Source: three-view drawing plus pictorial views. Frame: mm from the lowest corner of the part. Give positions to 0.01 mm unless a question says otherwise; leave off trailing zeros. Loops run counter-clockwise (first coordinate to the right, second up) from the corner with the lowest first, then second, coordinate; pieces in that order, holes last. Notation, with made-up numbers: (6.25, 35.5) - (24.25, 35.5) arc R33 ccw to (24.25, 73.5) - close; hole circle Ø1 at (45, 25.5). An arc over 180 degrees is marked (long way). One line per item, written item: value.
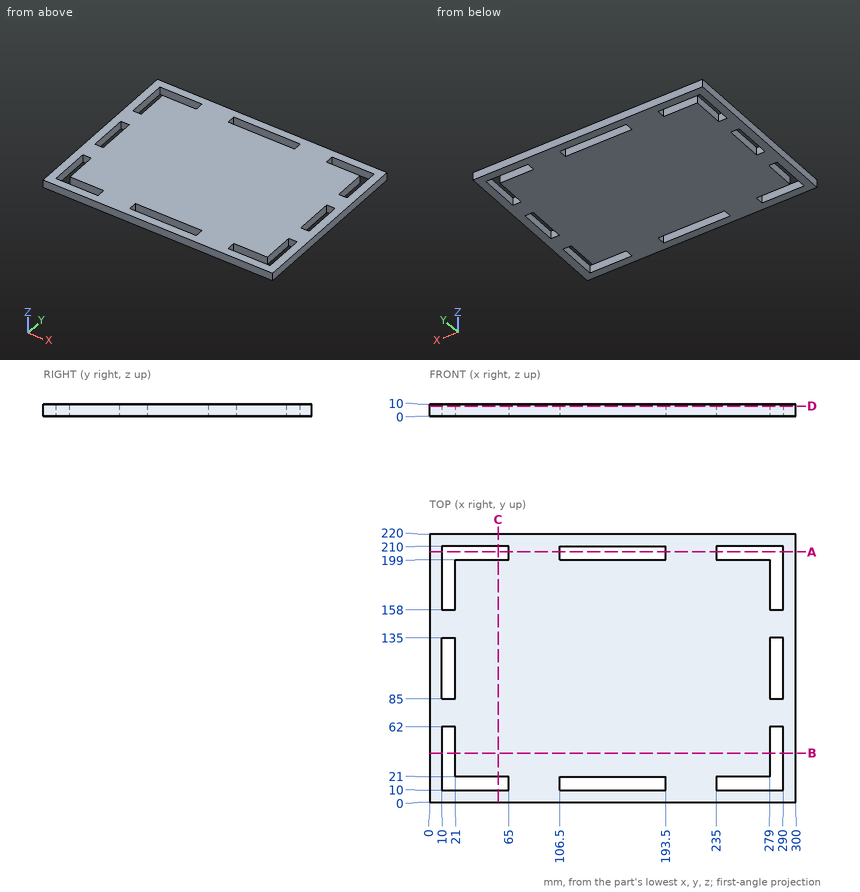
Item 1: Section C-C, the plane x = 56. Output: boundary loops of the cut face in (y, z), and give its area (3 significant figures).
Verdict:
outline: (0, 0) - (10, 0) - (10, 10) - (0, 10) - close; (21, 0) - (199, 0) - (199, 10) - (21, 10) - close; (210, 0) - (220, 0) - (220, 10) - (210, 10) - close
area: 1,980 mm^2
Item 2: Section D-D, the plane z = 8.25. Count the separate pieces of the cut face and the enclosed holes in it, and give its area (3 significant figures).
Verdict:
separate pieces: 1
enclosed holes: 8
area: 58,800 mm^2
Item 3: Material intervals for L1, parallel to X at y = 177, z = 9; L2, parallel to Y at x = 270, z = 8.75; L3, parallel to X at y = 13, z = 5, sorted ascending.
Verdict:
L1: x = 0 to 10, 21 to 279, 290 to 300
L2: y = 0 to 10, 21 to 199, 210 to 220
L3: x = 0 to 10, 65 to 106.5, 193.5 to 235, 290 to 300
Item 4: Section B-B, the plane y = 40.5. Output: boundary loops of the cut face in (x, z).
Verdict:
outline: (0, 0) - (10, 0) - (10, 10) - (0, 10) - close; (21, 0) - (279, 0) - (279, 10) - (21, 10) - close; (290, 0) - (300, 0) - (300, 10) - (290, 10) - close
Item 5: Section A-A, the plane y = 205.5. Output: boundary loops of the cut face in (x, z), and give its area (3 significant figures).
Verdict:
outline: (0, 0) - (10, 0) - (10, 10) - (0, 10) - close; (65, 0) - (106.5, 0) - (106.5, 10) - (65, 10) - close; (193.5, 0) - (235, 0) - (235, 10) - (193.5, 10) - close; (290, 0) - (300, 0) - (300, 10) - (290, 10) - close
area: 1,030 mm^2
